CAD build for the part. Positions are in the model's coordinates, mm. A direction names the side the tool comes from. Give positions to 0.01 mm unless a question says otherwise; leave off trailing zeros. Write each loop counter-clockwise with the first axis right and the second up, starting at its lowest first coordinate (ties: lowest second). Pieces come first, ordered by that corner, then holes. Notation, with made-up numbers: (15.25, 45.5) - (70.25, 45.5) arc R25 cw to (70.25, 66.5) - close; hole circle Ø3 at (-15, -19.5). An arc over 180 degrees is marked (long way). Answer as a JSON object with one key per item and string values.
from build123d import *

# Parameters (mm, degrees)
F0_R     = 14.2875
F0_R_2   = 6.35
F1_DEPTH = 7.112
F2_R     = 15.24
F3_DEPTH = 1.27
F4_R     = 6.35
F5_DEPTH = 25.4


with BuildPart() as f1:
    # F0 (on Front) → F1 (new body)
    with BuildSketch(Plane.XZ):
        with Locations((-66.254035, 44.382535)):
            Circle(F0_R)
        with Locations((-66.254035, 44.382535)):
            Circle(F0_R_2, mode=Mode.SUBTRACT)
    extrude(amount=F1_DEPTH)

    # F2 (on face) → F3 (join)
    with BuildSketch(Plane.XZ.offset(7.112)):
        with Locations((-66.254035, 44.382535)):
            Circle(F2_R)
    extrude(amount=-F3_DEPTH)

    # F4 (on face) → F5 (cut)
    with BuildSketch(Plane.XZ.offset(7.112)):
        with Locations((-66.254035, 44.382535)):
            Circle(F4_R)
    extrude(amount=-F5_DEPTH, mode=Mode.SUBTRACT)


solid = f1.part
Item 1: Flat gauge pins, fed straight in: P1, Ø2, axis at y = -4, z = 43.5, coming from the +X side; P2, Ø1.5, axis at y = -4.5, z = 54.5, coming from the -X side. Where does each tip first touch, or does it go through?
Entries:
{"P1": "x = -51.97", "P2": "x = -77.04"}
Item 2: Which spindle directions (+Z, -Z, +X, -X, +Y, -Y) get a long thin tool onto all of the face, cutting with end or side? Do faces 1 (the cylindrical face through (-68.11, -2.88, 58.55)), 2 (the cylindrical face through (-51.718, -6.486, 48.96)). Say none if no direction does.
Entries:
{"face 1": "+Y", "face 2": "+Y, -Y"}
Item 3: Cut at A-A (z = 44). Give the cut face in (x, y), and give its area (3 significant figures).
Entries:
{"outline": "(-81.49, -7.11) - (-72.59, -7.11) - (-72.59, 0) - (-80.54, 0) - (-80.54, -5.84) - (-81.49, -5.84) - close; (-59.92, -7.11) - (-51.02, -7.11) - (-51.02, -5.84) - (-51.97, -5.84) - (-51.97, 0) - (-59.92, 0) - close", "area": "115 mm2"}
Item 4: Probe line 1 (Z direction, x = -66.5, y = -5.5); line 2 (Z direction, x = -62.5, y = -2); line 3 (X direction, y = -5.25, z = 41). List the from-to ranges inside material, lowest first. Write a range as from..to.
Entries:
{"line 1": "30.1..38.04, 50.73..58.67", "line 2": "30.6..39.26, 49.5..58.17", "line 3": "-80.14..-71.63, -60.88..-52.37"}
Item 5: Cut at C-C (x = -73.5). Give the cut face in (y, z), and give its area (3 significant figures).
Entries:
{"outline": "(-7.11, 30.98) - (-5.84, 30.98) - (-5.84, 32.07) - (0, 32.07) - (0, 56.7) - (-5.84, 56.7) - (-5.84, 57.79) - (-7.11, 57.79) - close", "area": "178 mm2"}
Item 6: Cut at D-D (z = 37). Give the cut face in (x, y).
Entries:
{"outline": "(-79.59, -7.11) - (-52.92, -7.11) - (-52.92, -5.84) - (-54.02, -5.84) - (-54.02, 0) - (-78.49, 0) - (-78.49, -5.84) - (-79.59, -5.84) - close"}
Item 7: Cut at B-B (x = -63.5). Give the cut face in (y, z), and give its area (3 significant figures).
Entries:
{"outline": "(-7.11, 29.39) - (-5.84, 29.39) - (-5.84, 30.36) - (0, 30.36) - (0, 38.66) - (-7.11, 38.66) - close; (-7.11, 50.1) - (0, 50.1) - (0, 58.4) - (-5.84, 58.4) - (-5.84, 59.37) - (-7.11, 59.37) - close", "area": "120 mm2"}
